```python
from build123d import *

# Parameters (mm, degrees)
F0_R     = 8.5
F1_DEPTH = 10
F0_R_2   = 2
F2_DEPTH = 8
F0_R_3   = 1.5
F3_DEPTH = 1.5
F4_DEPTH = 10


with BuildPart() as f1:
    # F0 (on Front) → F1 (new body)
    with BuildSketch(Plane.XZ):
        with BuildLine():
            ThreePointArc((9.3658811475, -1.5906823473), (8.95, 0), (9.3658811475, 1.5906823473))
            ThreePointArc((9.3658811475, 1.5906823473), (0, 9.5), (-9.3658811475, 1.5906823473))
            ThreePointArc((-9.3658811475, 1.5906823473), (-9.0556887662, 0.8220747319), (-8.95, 0))
            ThreePointArc((-8.95, 0), (-9.0556887662, -0.8220747319), (-9.3658811475, -1.5906823473))
            ThreePointArc((-9.3658811475, -1.5906823473), (0, -9.5), (9.3658811475, -1.5906823473))
        make_face()
        Circle(F0_R, mode=Mode.SUBTRACT)
    extrude(amount=F1_DEPTH)

    # F0 (on Front) → F2 (join)
    with BuildSketch(Plane.XZ):
        with BuildLine():
            ThreePointArc((9.7654713115, -2.1530374044), (9.941194926, -1.082886625), (10, 0))
            ThreePointArc((10, 0), (9.941194926, 1.082886625), (9.7654713115, 2.1530374044))
            ThreePointArc((9.7654713115, 2.1530374044), (9.550712826, 1.8824923558), (9.3658811475, 1.5906823473))
            ThreePointArc((9.3658811475, 1.5906823473), (9.4664109065, 0.7981632347), (9.5, 0))
            ThreePointArc((9.5, 0), (9.4664109065, -0.7981632347), (9.3658811475, -1.5906823473))
            ThreePointArc((9.3658811475, -1.5906823473), (9.550712826, -1.8824923558), (9.7654713115, -2.1530374044))
        make_face()
        with BuildLine():
            ThreePointArc((9.7654713115, 2.1530374044), (9.941194926, 1.082886625), (10, 0))
            ThreePointArc((10, 0), (9.941194926, -1.082886625), (9.7654713115, -2.1530374044))
            ThreePointArc((9.7654713115, -2.1530374044), (13.3511476366, -3.0393024066), (15.45, 0))
            ThreePointArc((15.45, 0), (13.3511476366, 3.0393024066), (9.7654713115, 2.1530374044))
        make_face()
        with Locations((12.2, 0)):
            Circle(F0_R_2, mode=Mode.SUBTRACT)
        with BuildLine():
            ThreePointArc((9.3658811475, 1.5906823473), (9.550712826, 1.8824923558), (9.7654713115, 2.1530374044))
            ThreePointArc((9.7654713115, 2.1530374044), (0, 10), (-9.7654713115, 2.1530374044))
            ThreePointArc((-9.7654713115, 2.1530374044), (-9.550712826, 1.8824923558), (-9.3658811475, 1.5906823473))
            ThreePointArc((-9.3658811475, 1.5906823473), (0, 9.5), (9.3658811475, 1.5906823473))
        make_face()
        with BuildLine():
            ThreePointArc((-9.7654713115, -2.1530374044), (0, -10), (9.7654713115, -2.1530374044))
            ThreePointArc((9.7654713115, -2.1530374044), (9.550712826, -1.8824923558), (9.3658811475, -1.5906823473))
            ThreePointArc((9.3658811475, -1.5906823473), (0, -9.5), (-9.3658811475, -1.5906823473))
            ThreePointArc((-9.3658811475, -1.5906823473), (-9.550712826, -1.8824923558), (-9.7654713115, -2.1530374044))
        make_face()
        with BuildLine():
            ThreePointArc((-9.3658811475, 1.5906823473), (-9.550712826, 1.8824923558), (-9.7654713115, 2.1530374044))
            ThreePointArc((-9.7654713115, 2.1530374044), (-10, 0), (-9.7654713115, -2.1530374044))
            ThreePointArc((-9.7654713115, -2.1530374044), (-9.550712826, -1.8824923558), (-9.3658811475, -1.5906823473))
            ThreePointArc((-9.3658811475, -1.5906823473), (-9.5, 0), (-9.3658811475, 1.5906823473))
        make_face()
        with BuildLine():
            ThreePointArc((-9.7654713115, -2.1530374044), (-10, 0), (-9.7654713115, 2.1530374044))
            ThreePointArc((-9.7654713115, 2.1530374044), (-15.45, 0), (-9.7654713115, -2.1530374044))
        make_face()
        with Locations((-12.2, 0)):
            Circle(F0_R_2, mode=Mode.SUBTRACT)
    extrude(amount=F2_DEPTH)

    # F0 (on Front) → F3 (join)
    with BuildSketch(Plane.XZ):
        Circle(F0_R)
        with Locations((-4.5, 0)):
            Circle(F0_R_3, mode=Mode.SUBTRACT)
        with Locations((4.5, 0)):
            Circle(F0_R_3, mode=Mode.SUBTRACT)
    extrude(amount=F3_DEPTH)

    # F0 (on Front) → F4 (join)
    with BuildSketch(Plane.XZ):
        with BuildLine():
            ThreePointArc((9.5, 0), (9.4664109065, 0.7981632347), (9.3658811475, 1.5906823473))
            ThreePointArc((9.3658811475, 1.5906823473), (8.95, 0), (9.3658811475, -1.5906823473))
            ThreePointArc((9.3658811475, -1.5906823473), (9.4664109065, -0.7981632347), (9.5, 0))
        make_face()
        with BuildLine():
            ThreePointArc((-8.95, 0), (-9.0556887662, 0.8220747319), (-9.3658811475, 1.5906823473))
            ThreePointArc((-9.3658811475, 1.5906823473), (-9.5, 0), (-9.3658811475, -1.5906823473))
            ThreePointArc((-9.3658811475, -1.5906823473), (-9.0556887662, -0.8220747319), (-8.95, 0))
        make_face()
    extrude(amount=F4_DEPTH)


solid = f1.part
```
Design review of the part built by this model. Coordinates are the model's own, in mm. A direction names the side the tool comes from. Give positions to 0.01 mm unless a question says otherwise; leave off trailing zeros. Order: outer loops, then holes, each group sorted by start corner. A loop starts at its lowest first (then second) coordinate and runs counter-clockwise, first axis right, second up. Notation, with made-up numbers: (54.5, -11.5) - (109.5, -11.5) arc R28 cw to (109.5, 16.5) - close; hole circle Ø9 at (41, -40). An arc over 180 degrees is marked (long way). Use a Markdown table: item, result. Add a question column.
(1) Add section B-B on y = -2. Give the boundary of the cut face in (x, z), then the cut area to 3 significant figures.
(2) Add section A-A on x = -12.2. Give the boundary of the cut face in (y, z), then the cut area to 3 significant figures.
(3) Clearance check with flat-ended pins moving along their axes: P1, Ø2, axis at x = 5.5, y = -4.5, coming from the -Z side; P2, Ø10, axis at x = 1.5, z = -4.5, coming from the -Y side; P3, Ø3.5, axis at x = -12.2, z = 0, coming from the -Y side; P4, Ø2, axis at x = 5, y = -6, coming from the -Z side. State where each tip first meets the part, or that it passes through.
(4) Machinability: for faces 3 (the face through (4.57, -5.69, 7.167)), 4 (the face through (14.108, -3.944, 0.601)), which of the approach directions +Z, -Z, +X, -X, +Y, -Y give a long, thin tool a straight path to every point of the face, cutting with its end or side? Answer none if there is none.
(5) Wall thickness on probe 1 along X at (y, z) = (-7.5, -2.75); probe 2 along X at (y, z) = (-9, -0.25); probe 3 along Z at (x, y) = (-12.2, -3): over which ranges is each line inside the solid? List them lowest first. Write a range as [from, to].
(6) Mouldability with a two-part tool opening along Z and no side actions: class faces 1 (the face through (-2.2, -10, -8.4)), 2 (the face through (5.886, -0.74, -0.575)) as +Z half, -Z half, draft (parallel to the pull), parting line (faces both ways), or undercut.
(7) Add section D-D on x = 0. Give the boundary of the cut face in (y, z).
(8) Add section C-C on y = -8.75. Give the boundary of the cut face in (x, z), then the cut area to 3 significant figures.
Report:
| question | item | result |
|---|---|---|
| 1 | outline | (-9.77, -2.15) arc R10 ccw to (9.77, -2.15) arc R3.25 ccw (long way) to (9.77, 2.15) arc R10 ccw to (-9.77, 2.15) arc R3.25 ccw (long way) to start; hole circle Ø4 at (-12.2, 0); hole circle Ø17 at (0, 0); hole circle Ø4 at (12.2, 0) |
| 1 | area | 122 mm² |
| 2 | outline | (-8, -3.25) - (0, -3.25) - (0, -2) - (-8, -2) - close; (-8, 2) - (0, 2) - (0, 3.25) - (-8, 3.25) - close |
| 2 | area | 20.0 mm² |
| 3 | P1 | stops at z = -8.93 |
| 3 | P2 | stops at y = -10 |
| 3 | P3 | passes through |
| 3 | P4 | stops at z = -9.17 |
| 4 | face 3 | -Y |
| 4 | face 4 | +Y, -Y |
| 5 | probe 1 | x = [-13.93, -10.47], [-9.61, -8.04], [8.04, 9.61], [10.47, 13.93] |
| 5 | probe 2 | x = [-9.5, -8.5], [8.5, 9.5] |
| 5 | probe 3 | z = [-3.25, -2], [2, 3.25] |
| 6 | face 1 | draft |
| 6 | face 2 | undercut |
| 7 | outline | (-10, -9.5) - (-8, -9.5) - (-8, -10) - (0, -10) - (0, 10) - (-8, 10) - (-8, 9.5) - (-10, 9.5) - (-10, 8.5) - (-1.5, 8.5) - (-1.5, -8.5) - (-10, -8.5) - close |
| 8 | outline | circle Ø19 at (0, 0); hole circle Ø17 at (0, 0) |
| 8 | area | 56.5 mm² |
